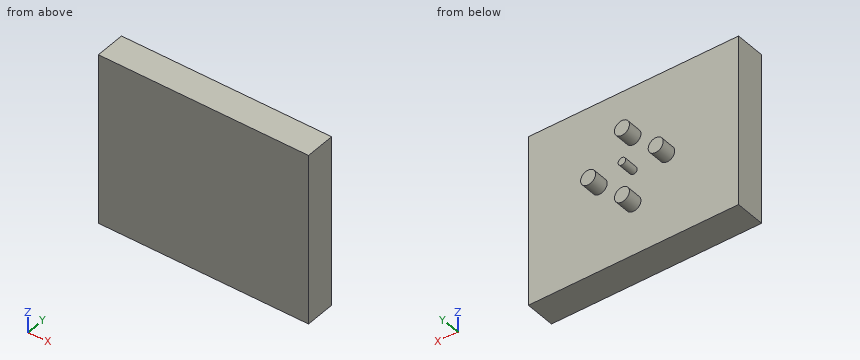
from build123d import *

# Parameters (mm, degrees)
F0_W     = 177.718074
F0_H     = 144.534186
F1_DEPTH = 25.4
F3_R     = 3.175
F4_DEPTH = 12.7
F5_R     = 6.35
F6_DEPTH = 12.7


with BuildPart() as f1:
    # F0 (on Front) → F1 (new body)
    with BuildSketch(Plane.XZ):
        Rectangle(F0_W, F0_H)
    extrude(amount=F1_DEPTH)

    # F3 (on face) → F4 (join)
    with BuildSketch(Plane(origin=(0, 0, 0), x_dir=(-1, 0, 0), z_dir=(0, 1, 0))):
        Circle(F3_R)
    extrude(amount=F4_DEPTH)

    # F5 (on face) → F6 (join)
    with BuildSketch(Plane(origin=(0, 0, 0), x_dir=(-1, 0, 0), z_dir=(0, 1, 0))):
        with Locations((-28.575, 0)):
            Circle(F5_R)
        with Locations((0, 28.575)):
            Circle(F5_R)
        with Locations((28.575, 0)):
            Circle(F5_R)
        with Locations((0, -28.575)):
            Circle(F5_R)
    extrude(amount=F6_DEPTH)


solid = f1.part
Build history of the part. All positions in model axes, mm. Round coordinates to 2 decimals unless told otherwise and drop trailing zeros. Write each loop counter-clockwise with the first axis right and the second up, starting at its lowest first coordinate (ties: lowest second). Pieces come first, ordered by that corner, then holes. Notation, with made-up numbers: M 10.5,88 L 35.5,88 A29 ccw 35.5,122 Z; hole C -13.5,-10 d10. An arc over 180 degrees is marked long. Answer as a JSON object with one key per item and string values. Group by question number.
(1) Cut at B-B (x = 0). Give the cut face in (y, z) (3 decimals).
(2) Flat gauge pins, fed straight in: pin 1 (10 mm diameter, centred on x = -1, z = 57.5, fed in from +Y); pin 2 (10 mm diameter, centred on x = -20, y = 8, fed in from -Z). Where does each tip first touch, or does it go through?
(3) Drill centre lines: L1, parallel to Y at x = -3.5, z = -14.5; L2, parallel to X at y = 11, z = 28.5; L3, parallel to X at y = 7.5, z = 23. Where is each one in solid material? Low to high.
(4) Cut at C-C (y = 5.5). Give the cut face in (x, z) (3 decimals), and give its area (3 significant figures).
(5) Cut at D-D (x = 33). Give the cut face in (y, z), and give its area (3 significant figures).
(6) Cut at A-A (z = 0). Give the cut face in (x, y) (3 decimals).
Responses:
{
 "1": {"outline": "M -25.4,-72.267 L 0,-72.267 L 0,-34.925 L 12.7,-34.925 L 12.7,-22.225 L 0,-22.225 L 0,-3.175 L 12.7,-3.175 L 12.7,3.175 L 0,3.175 L 0,22.225 L 12.7,22.225 L 12.7,34.925 L 0,34.925 L 0,72.267 L -25.4,72.267 Z"},
 "2": {"pin 1": "stops at y = 0", "pin 2": "stops at z = -5.25"},
 "3": {"L1": "y = -25.4 to 0", "L2": "x = -6.35 to 6.35", "L3": "x = -3.04 to 3.04"},
 "4": {"outline": "C -28.575,0 d12.7; C 0,-28.575 d12.7; C 0,28.575 d12.7; C 0,0 d6.35; C 28.575,0 d12.7", "area": "538 mm2"},
 "5": {"outline": "M -25.4,-72.27 L 0,-72.27 L 0,-4.55 L 12.7,-4.55 L 12.7,4.55 L 0,4.55 L 0,72.27 L -25.4,72.27 Z", "area": "3,790 mm2"},
 "6": {"outline": "M -88.859,-25.4 L 88.859,-25.4 L 88.859,0 L 34.925,0 L 34.925,12.7 L 22.225,12.7 L 22.225,0 L 3.175,0 L 3.175,12.7 L -3.175,12.7 L -3.175,0 L -22.225,0 L -22.225,12.7 L -34.925,12.7 L -34.925,0 L -88.859,0 Z"}
}
